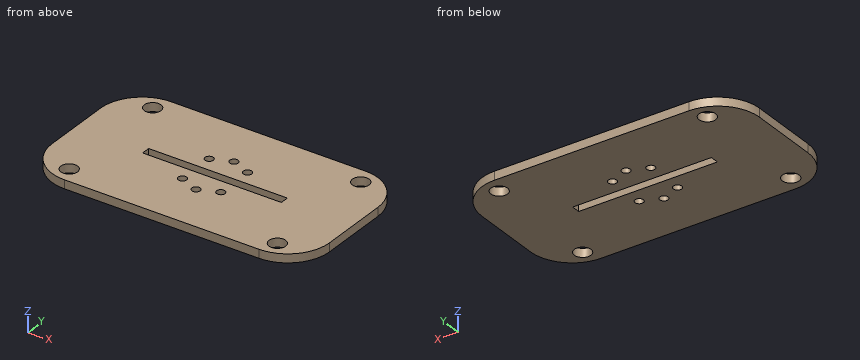
from build123d import *

# Parameters (mm, degrees)
SKETCH1_W           = 100
SKETCH1_H           = 55
SKETCH1_R           = 3
SKETCH1_W_2         = 50
SKETCH1_H_2         = 3.1
BOSS_EXTRUDE1_DEPTH = 3.1
SKETCH2_R           = 1.5
CUT_EXTRUDE1_DEPTH  = 4.1
FILLET1_R           = 15


with BuildPart() as part:
    # Sketch1 → Boss-Extrude1 (new body)
    with BuildSketch(Plane.XY):
        Rectangle(SKETCH1_W, SKETCH1_H)
        with Locations((37.5, 21.55)):
            Circle(SKETCH1_R, mode=Mode.SUBTRACT)
        with Locations((-37.5, 21.55)):
            Circle(SKETCH1_R, mode=Mode.SUBTRACT)
        with Locations((-37.5, -21.55)):
            Circle(SKETCH1_R, mode=Mode.SUBTRACT)
        with Locations((37.5, -21.55)):
            Circle(SKETCH1_R, mode=Mode.SUBTRACT)
        Rectangle(SKETCH1_W_2, SKETCH1_H_2, mode=Mode.SUBTRACT)
    extrude(amount=BOSS_EXTRUDE1_DEPTH)

    # Sketch2 → Cut-Extrude1 (cut, through all)
    with BuildSketch(Plane.XY.offset(3.1)):
        with Locations((-6.914797213, 6.914797213)):
            Circle(SKETCH2_R)
        with Locations((0, 9.779)):
            Circle(SKETCH2_R)
        with Locations((6.914797213, 6.914797213)):
            Circle(SKETCH2_R)
        with Locations((9.779, 0)):
            Circle(SKETCH2_R)
        with Locations((6.914797213, -6.914797213)):
            Circle(SKETCH2_R)
        with Locations((0, -9.779)):
            Circle(SKETCH2_R)
        with Locations((-6.914797213, -6.914797213)):
            Circle(SKETCH2_R)
        with Locations((-9.779, 0)):
            Circle(SKETCH2_R)
    extrude(amount=-CUT_EXTRUDE1_DEPTH, mode=Mode.SUBTRACT)

    # Fillet1
    fillet1_edges = [part.edges().sort_by_distance(p)[0] for p in [
        (50, -27.5, 1.55),
        (-50, -27.5, 1.55),
        (-50, 27.5, 1.55),
        (50, 27.5, 1.55),
    ]]
    fillet(fillet1_edges, radius=FILLET1_R)


solid = part.part
Work out the finished part from the listing and answer in its coordinate system (mm). Give positions to 0.01 mm unless a question says otherwise; leave off trailing zeros. Loops run counter-clockwise (first coordinate to the right, second up) from the corner with the lowest first, then second, coordinate; pieces in that order, holes last. Notation, with made-up numbers: (11.25, 26.5) - (21.25, 26.5) arc R27 cw to (21.25, 65.5) - close; hole circle Ø6 at (-32.5, -11). An arc over 180 degrees is marked (long way). Answer in a Markdown table with one row per item. Add a question column.
Q1. Consider line 1 along Y through (x, z) = (-7, 1.1); line 2 along Y through (x, z) = (0, 1.65); line 3 along Y through (x, z) = (23.5, 0.7). Determine where each line is inside the solid, lowest interval first.
Q2. The part is cut by section A-A (x = -15). Determine the outline of the cut face in (y, z), and give its area (3 significant figures).
Q3. The part is cut by section C-C (z = 1.9). State how many separate pieces and enclosed holes the cut face has, and give its area (3 significant figures).
Q4. The part is cut by section D-D (y = -21.55). Determine the outline of the cut face in (x, z).
Q5. The part is cut by section B-B (x = 38). Determine the outline of the cut face in (y, z).
Solution:
| question | item | result |
|---|---|---|
| 1 | line 1 | y = -27.5 to -8.41, -5.42 to -1.55, 1.55 to 5.42, 8.41 to 27.5 |
| 1 | line 2 | y = -27.5 to -11.28, -8.28 to -1.55, 1.55 to 8.28, 11.28 to 27.5 |
| 1 | line 3 | y = -27.5 to -1.55, 1.55 to 27.5 |
| 2 | outline | (-27.5, 0) - (-1.55, 0) - (-1.55, 3.1) - (-27.5, 3.1) - close; (1.55, 0) - (27.5, 0) - (27.5, 3.1) - (1.55, 3.1) - close |
| 2 | area | 161 mm² |
| 3 | separate pieces | 1 |
| 3 | enclosed holes | 11 |
| 3 | area | 5,000 mm² |
| 4 | outline | (-46.96, 0) - (-40.5, 0) - (-40.5, 3.1) - (-46.96, 3.1) - close; (-34.5, 0) - (34.5, 0) - (34.5, 3.1) - (-34.5, 3.1) - close; (40.5, 0) - (46.96, 0) - (46.96, 3.1) - (40.5, 3.1) - close |
| 5 | outline | (-27.2, 0) - (-24.51, 0) - (-24.51, 3.1) - (-27.2, 3.1) - close; (-18.59, 0) - (18.59, 0) - (18.59, 3.1) - (-18.59, 3.1) - close; (24.51, 0) - (27.2, 0) - (27.2, 3.1) - (24.51, 3.1) - close |
